Autodesk Inventor part; units mm, degrees
ref_plane "YZ Plane" through (0, 0, 0) normal (1, 0, 0) x (0, 1, 0)
ref_plane "XZ Plane" through (0, 0, 0) normal (0, 1, 0) x (-1, 0, 0)
ref_plane "XY Plane" through (0, 0, 0) normal (0, 0, 1) x (1, 0, 0)
sketch "Sketch1" plane through (0, 0, 0) normal (1, 0, 0) x (0, 1, 0)
  line L0 (11.25, 0) -> (-11.25, 0) construction
  line L1 (-11.25, 12.5) -> (11.25, 12.5)
  line L2 (11.25, 0) -> (-11.25, 0)
  line L3 (-11.25, 12.5) -> (-11.25, 16)
  line L4 (-11.25, 16) -> (11.25, 16)
  line L5 (11.25, 16) -> (11.25, 12.5)
  line L6 (-11.25, 16) -> (3.75, 16)
  line L7 (3.75, 16) -> (3.75, 18)
  line L8 (3.75, 18) -> (-11.25, 18)
  line L9 (-11.25, 18) -> (-11.25, 16)
  line L10 (-11.25, 18) -> (-8.25, 18)
  line L11 (-8.25, 18) -> (-8.25, 42.5)
  line L12 (-8.25, 42.5) -> (-11.25, 42.5)
  line L13 (-11.25, 42.5) -> (-11.25, 18)
  point P0 (0, 0)
  dimension "d0" = 12.5
  dimension "d1" = 0
  dimension "d2" = 22.5
  dimension "d3" = 16
  dimension "d6" = 18
  dimension "d7" = 7.5
  dimension "d8" = 42.5
  dimension "d10" = 11.25
  dimension "d11" = 19.5
revolve "Revolution1" add sketch "Sketch1" angle 360 about axis through (0, 11.25, 0) along (0, -1, 0)
equation "\"d2\" = d4 + d5"
equation "\"d5\" = d4"
Could you check a few things on this model? Use its own coordinates, in mm. A direction names the side the tool comes from. Round coordinates to 2 decimals unless told otherwise and drop trailing zeros. Write each loop counter-clockwise with the first axis right and the second up, starting at its lowest first coordinate (ties: lowest second). Pieces come first, ordered by that corner, then holes. Notation, with made-up numbers: (30, 64.25) - (45, 64.25) arc R30 ccw to (45, 103.25) - close; hole circle Ø6 at (38.25, 72). An arc over 180 degrees is marked (long way). Use a Markdown table: item, result.
Q1. I want a section at D-D (x = -15). List the corners of the cut face in (y, z) for me, plus the area to 3 significant figures.
Output values:
| item | result |
|---|---|
| outline | (-11.25, -39.76) - (-8.25, -39.76) - (-8.25, -9.95) - (3.75, -9.95) - (3.75, -5.57) - (11.25, -5.57) - (11.25, 5.57) - (3.75, 5.57) - (3.75, 9.95) - (-8.25, 9.95) - (-8.25, 39.76) - (-11.25, 39.76) - close |
| area | 561 mm2 |
Q2. Thinking about a two-plate mould opening in X: for faces 1 (the cylindrical face through (3.755, 0.158, 11.923)), 2 (the cylindrical face through (25.861, -9.771, -33.727)), 3 (the flat face through (11, 3.75, -12)), which applies, released by +X, released by -X, zero draft, split by the parting line, or undercut?
Output values:
| item | result |
|---|---|
| face 1 | undercut |
| face 2 | split by the parting line |
| face 3 | zero draft |
Q3. Please list where these lines run through material, in increasing order: L1, parallel to X at y = 5, z = 0; L2, parallel to Z at x = 0, y = -0.75.
Output values:
| item | result |
|---|---|
| L1 | -16 to -12.5, 12.5 to 16 |
| L2 | -18 to -12.5, 12.5 to 18 |
Q4. For faces 4 (the cylindrical face through (-17.847, -2.334, -2.343)), 5 (the flat face through (9, -11.25, 9)), which set-ups out of +Z, -Z, +X, -X, +Y, -Y let a thin tool reach every point of the face, with its end or its side?
Output values:
| item | result |
|---|---|
| face 4 | +Y |
| face 5 | +Z, -Z, +X, -X, -Y |
Q5. I want a section at C-C (y = -9.5). List the corners of the cut face in (x, z) for me, plus the area to 3 significant figures.
Output values:
| item | result |
|---|---|
| outline | circle Ø85 at (0, 0); hole circle Ø25 at (0, 0) |
| area | 5,180 mm2 |
Q6. I want a section at B-B (z = 0). List the corners of the cut face in (x, y) for me, plus the area to 4 significant figures.
Output values:
| item | result |
|---|---|
| outline | (-42.5, -11.25) - (-12.5, -11.25) - (-12.5, 11.25) - (-16, 11.25) - (-16, 3.75) - (-18, 3.75) - (-18, -8.25) - (-42.5, -8.25) - close; (12.5, -11.25) - (42.5, -11.25) - (42.5, -8.25) - (18, -8.25) - (18, 3.75) - (16, 3.75) - (16, 11.25) - (12.5, 11.25) - close |
| area | 364.5 mm2 |
Q7. For pin 1 (1 mm diameter, centred on x = -1.5, z = 26.5, fed in from +Y); pin 2 (5 mm diameter, centred on y = -7.5, z = 26.5, fed in from +X); pin 3 (4 mm diameter, centred on x = -9, y = -3.5, fed in from -Z); pin 4 (11 mm diameter, centred on x = -1.5, z = -4.5, fed in from +Y), each with a flat end and sliding along its axis, tell me the tip position at first contact or that it passes through.
Output values:
| item | result |
|---|---|
| pin 1 | y = -8.25 |
| pin 2 | x = 35 |
| pin 3 | z = -16.58 |
| pin 4 | through |
Q8. I want a section at A-A (x = 0). List the corners of the cut face in (y, z) for me, plus the area to 4 significant figures.
Output values:
| item | result |
|---|---|
| outline | (-11.25, -42.5) - (-8.25, -42.5) - (-8.25, -18) - (3.75, -18) - (3.75, -16) - (11.25, -16) - (11.25, -12.5) - (-11.25, -12.5) - close; (-11.25, 12.5) - (11.25, 12.5) - (11.25, 16) - (3.75, 16) - (3.75, 18) - (-8.25, 18) - (-8.25, 42.5) - (-11.25, 42.5) - close |
| area | 364.5 mm2 |
